Autodesk Fusion 360 part; units mm, degrees
sketch "Sketch1" plane through (0, 0, 0) normal (0, 0, 1) x (1, 0, 0)
  line L0 (40, 22) -> (-40, 22)
  line L1 (-40, 22) -> (-40, -22)
  line L2 (-40, -22) -> (40, -22)
  line L3 (40, -22) -> (40, 22)
  line L4 (40, 22) -> (-40, -22) construction
  line L5 (-40, 22) -> (40, -22) construction
  line L6 (33, 15) -> (-33, 15)
  line L7 (-33, 15) -> (-33, -15)
  line L8 (-33, -15) -> (33, -15)
  line L9 (33, -15) -> (33, 15)
  line L10 (33, 15) -> (-33, -15) construction
  line L11 (-33, 15) -> (33, -15) construction
  line L12 (23, 11) -> (-23, 11)
  line L13 (-23, 11) -> (-23, -11)
  line L14 (-23, -11) -> (23, -11)
  line L15 (23, -11) -> (23, 11)
  line L16 (23, 11) -> (-23, -11) construction
  line L17 (-23, 11) -> (23, -11) construction
  line L18 (-40, 18.1224) -> (40, 18.1224) construction
  line L19 (-40, -17.8776) -> (40, -17.8776) construction
  line L20 (-36, 22) -> (-36, -22) construction
  line L21 (36, 22) -> (36, -22) construction
  circle A0 centre (-36, 18.1224) radius 1.8
  circle A1 centre (36, 18.1224) radius 1.8
  circle A2 centre (-36, -17.8776) radius 1.8
  circle A3 centre (36, -17.8776) radius 1.8
  line L22 (-20, 22) -> (-20, -22) construction
  line L23 (0, 22) -> (0, -22) construction
  line L24 (20, 22) -> (20, -22) construction
  dimension "d1" = 80
  dimension "d2" = 44
  dimension "d3" = 66
  dimension "d4" = 30
  dimension "d5" = 46
  dimension "d6" = 22
  dimension "d7" = 36
  dimension "d8" = 72
  dimension "d9" = 4
  dimension "d10" = 3.6
  dimension "d11" = 3.6
  dimension "d12" = 3.6
  dimension "d13" = 3.6
  dimension "d14" = 16
sketch "Sketch2" plane through (0, 0, 0) normal (0, 0, 1) x (1, 0, 0)
extrude "Extrude1" add sketch "Sketch1" along normal blind 3 contours L6 L7 L8 L9
extrude "Extrude2" add sketch "Sketch1" along normal blind 6 contours L0 L1 L2 L3
fillet "Fillet1" radius 11 1 edges at (-23, 11, 1.5)
fillet "Fillet2" radius 11 1 edges at (23, 11, 1.5)
fillet "Fillet3" radius 11 1 edges at (23, -11, 1.5)
fillet "Fillet4" radius 11 1 edges at (-23, -11, 1.5)
sketch "Sketch3" plane through (0, 0, 0) normal (0, 0, 1) x (1, 0, 0)
  circle A0 centre (-20, 11) radius 1.6
  circle A1 centre (-20, -11) radius 1.6
  line L0 (0, 22) -> (0, -22)
  circle A2 centre (20, 11) radius 1.6
  circle A3 centre (20, -11) radius 1.6
  dimension "d29" = 3.2
  dimension "d30" = 3.2
extrude "Extrude3" cut sketch "Sketch3" along normal blind 12 contours A3
extrude "Extrude4" cut sketch "Sketch3" along normal blind 6 contours A2
extrude "Extrude5" cut sketch "Sketch3" along normal blind 8 contours A1
extrude "Extrude6" cut sketch "Sketch3" along normal blind 8 contours A0
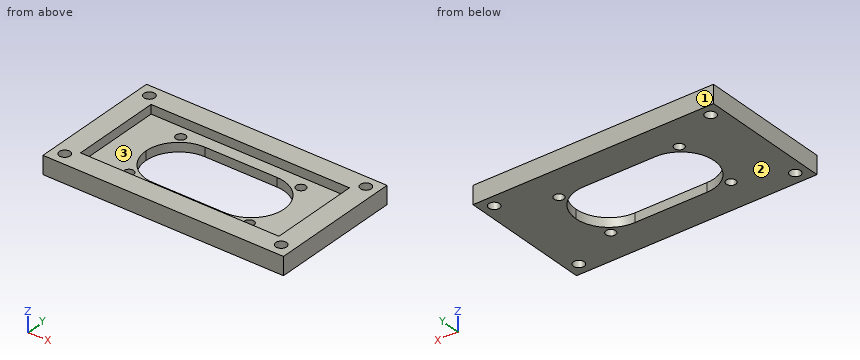
For this review, take the finished solid that the model builds, in its own axes (mm). Face numbers are marked on the shaded views. Round coordinates to 2 decimals unless told otherwise and drop trailing zeros. Loops run counter-clockwise (first coordinate to the right, second up) from the corner with the lowest first, then second, coordinate; pieces in that order, holes last. Notation, with made-up numbers: (83, -17) - (88, -17) arc R21 cw to (88, 16) - close; hole circle Ø2 at (57.25, 58). An arc over 180 degrees is marked (long way). Put each result on its own line as item: value. Start each with the question number.
1. Consider section A-A on x = 36. State the section outline as (y, z) points, plus the area to 3 significant figures.
2. For probe 1 along Y at (x, z) = (-36, 3.8); probe 2 along Y at (x, z) = (-0.5, 3.95); probe 3 along Y at (x, z) = (7.5, 0.7), list the stretches that pass through material, from the lowest coordinate up. Write a range as [from, to].
3. Consider section D-D on x = -20. State the section outline as (y, z) points, plus the area to 3 significant figures.
4. Mouldability with a two-part tool opening along Z and no side actions: class the marked faces 1, 2 and 3 as +Z half, -Z half, draft (parallel to the pull), parting line (faces both ways), or undercut.
5. Consider section B-B on x = 11. State the section outline as (y, z) points, plus the area to 3 significant figures.
6. Consider section C-C on z = 3.95. State the section outline as (x, y) points.
7. Insertion check: P1, Ø1.9, axis at x = 20, y = -11, coming from the +Z side. The pin has a flat end and moves straight along its axis. Give the tip position at first contact, or say it passes through.
Result sheet:
1. outline: (-22, 0) - (-19.68, 0) - (-19.68, 6) - (-22, 6) - close; (-16.08, 0) - (16.32, 0) - (16.32, 6) - (-16.08, 6) - close; (19.92, 0) - (22, 0) - (22, 6) - (19.92, 6) - close
1. area: 221 mm^2
2. probe 1: [-22, -19.68], [-16.08, 16.32], [19.92, 22]
2. probe 2: [-22, -15], [15, 22]
2. probe 3: [-22, -11], [11, 22]
3. outline: (-22, 0) - (-12.6, 0) - (-12.6, 3) - (-15, 3) - (-15, 6) - (-22, 6) - close; (-9.4, 0) - (-7.55, 0) - (-7.55, 3) - (-9.4, 3) - close; (7.55, 0) - (9.4, 0) - (9.4, 3) - (7.55, 3) - close; (12.6, 0) - (22, 0) - (22, 6) - (15, 6) - (15, 3) - (12.6, 3) - close
3. area: 109 mm^2
4. face 1: draft
4. face 2: -Z half
4. face 3: +Z half
5. outline: (-22, 0) - (-11, 0) - (-11, 3) - (-15, 3) - (-15, 6) - (-22, 6) - close; (11, 0) - (22, 0) - (22, 6) - (15, 6) - (15, 3) - (11, 3) - close
5. area: 108 mm^2
6. outline: (-40, -22) - (40, -22) - (40, 22) - (-40, 22) - close; hole circle Ø3.6 at (-36, -17.88); hole circle Ø3.6 at (-36, 18.12); hole (-33, -15) - (33, -15) - (33, 15) - (-33, 15) - close; hole circle Ø3.6 at (36, -17.88); hole circle Ø3.6 at (36, 18.12)
7. P1: through
